```python
from build123d import *

# Parameters (mm, degrees)
SKETCH1_W               = 72
SKETCH1_H               = 47
BOSS_EXTRUDE1_DEPTH     = 2
SKETCH2_R               = 1.75
CUT_EXTRUDE1_DEPTH      = 3
CUT_EXTRUDE1_DEPTH_BACK = 1


with BuildPart() as part:
    # Sketch1 → Boss-Extrude1 (new body)
    with BuildSketch(Plane.XY):
        Rectangle(SKETCH1_W, SKETCH1_H)
    extrude(amount=BOSS_EXTRUDE1_DEPTH)

    # Sketch2 → Cut-Extrude1 (cut, two sides)
    with BuildSketch(Plane.XY) as cut_extrude1_sk:
        with Locations((-32.75, 20.25)):
            Circle(SKETCH2_R)
        with Locations((32.75, 20.25)):
            Circle(SKETCH2_R)
        with Locations((32.75, -20.25)):
            Circle(SKETCH2_R)
        with Locations((-32.75, -20.25)):
            Circle(SKETCH2_R)
    extrude(amount=CUT_EXTRUDE1_DEPTH, mode=Mode.SUBTRACT)
    extrude(cut_extrude1_sk.sketch, amount=-CUT_EXTRUDE1_DEPTH_BACK, mode=Mode.SUBTRACT)


solid = part.part
```
Can you work these out from the model? Positions are in its coordinate system, mm. Coordinates: 2 decimals unless noted, no trailing zeros. Write each loop counter-clockwise with the first axis right and the second up, starting at its lowest first coordinate (ties: lowest second). Pieces come first, ordered by that corner, then holes. Notation, with made-up numbers: M 70.5,23 L 84.5,23 A20 cw 84.5,55 Z; hole C 18.5,61 d5. An arc over 180 degrees is marked long. Write item = value, one per line. Start each with the question number.
Q1. I'm going to push a flat-ended pin straight in: pin 1 (3 mm diameter, centred on x = 32.75, y = -20.25, fed in from +Z). Where does the tip first touch, or does it pass through?
Q2. Thinking about a two-plate mould opening in X: for faces 1 (the face through (-1, -23.5, 1)), 2 (the face through (-34.04, -19.07, 0.99)), 3 (the face through (-36, 0, 1)), which applies, released by +X, released by -X, zero draft, split by the parting line, or undercut?
Q3. If we section it at B-B, the plane y = 20.25: Write out the boundary of the cut face in (x, z).
Q4. If I drill on L1, parallel to X at y = -20.25, z = 0.45; L2, parallel to Y at x = -32.75, z = 1.6, over which ranges is the centre line in solid material (lowest first)? Write a range as [from, to].
Q5. If we section it at A-A, the plane x = -32.75: Write out the boundary of the cut face in (y, z), then the cut area to 3 significant figures.
Check sheet entries:
q1.pin_1 = through
q2.face_1 = zero draft
q2.face_2 = undercut
q2.face_3 = released by -X
q3.outline = M -36,0 L -34.5,0 L -34.5,2 L -36,2 Z; M -31,0 L 31,0 L 31,2 L -31,2 Z; M 34.5,0 L 36,0 L 36,2 L 34.5,2 Z
q4.L1 = [-36, -34.5], [-31, 31], [34.5, 36]
q4.L2 = [-23.5, -22], [-18.5, 18.5], [22, 23.5]
q5.outline = M -23.5,0 L -22,0 L -22,2 L -23.5,2 Z; M -18.5,0 L 18.5,0 L 18.5,2 L -18.5,2 Z; M 22,0 L 23.5,0 L 23.5,2 L 22,2 Z
q5.area = 80.0 mm²
